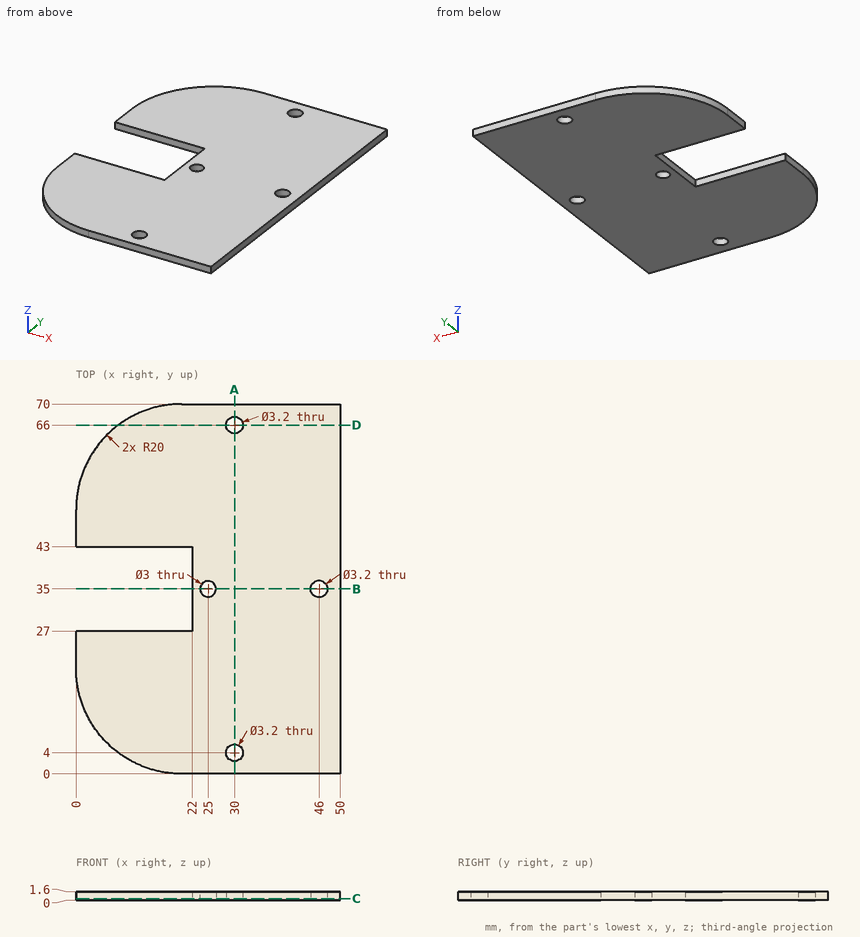
Study the drawing (mm; zero at the part's minimum x, y, z) and answer. Round coordinates to 2 decimals unless told otherwise and drop trailing zeros. Loops run counter-clockwise (first coordinate to the right, second up) from the corner with the lowest first, then second, coordinate; pieces in that order, holes last.
Q1. Section B-B, the plane y = 35 is taken. Determine the outline of the cut face in (x, z), then the cut area to 3 significant figures.
Q2. Section D-D, the plane y = 66 is taken. Determine the outline of the cut face in (x, z).
Q3. Section A-A, the plane x = 30 is taken. Determine the outline of the cut face in (y, z), then the cut area to 3 significant figures.
Q4. Find the intervals of material crossed by line 1 (Y direction, x = 30, z = 0.4); line 2 (Y direction, x = 19.5, z = 0.9); line 3 (X direction, y = 34, z = 1), in increasing order.
Q5. Section C-C, the plane z = 0.3 is taken. Determine the outline of the cut face in (x, y).
Q6. Given pin 1 Ø1.8 at (x, y) = (25, 35) entering from -Z, flat-ended and moving along its own axis, determine where the tip first touches the part or whether it passes through.
Completed:
1. outline: (22, 0) - (23.5, 0) - (23.5, 1.6) - (22, 1.6) - close; (26.5, 0) - (44.4, 0) - (44.4, 1.6) - (26.5, 1.6) - close; (47.6, 0) - (50, 0) - (50, 1.6) - (47.6, 1.6) - close
1. area: 34.9 mm2
2. outline: (8, 0) - (28.4, 0) - (28.4, 1.6) - (8, 1.6) - close; (31.6, 0) - (50, 0) - (50, 1.6) - (31.6, 1.6) - close
3. outline: (0, 0) - (2.4, 0) - (2.4, 1.6) - (0, 1.6) - close; (5.6, 0) - (64.4, 0) - (64.4, 1.6) - (5.6, 1.6) - close; (67.6, 0) - (70, 0) - (70, 1.6) - (67.6, 1.6) - close
3. area: 102 mm2
4. line 1: y = 0 to 2.4, 5.6 to 64.4, 67.6 to 70
4. line 2: y = 0.01 to 27, 43 to 69.99
4. line 3: x = 22 to 23.88, 26.12 to 44.75, 47.25 to 50
5. outline: (0, 20) arc R20 ccw to (20, 0) - (50, 0) - (50, 70) - (20, 70) arc R20 ccw to (0, 50) - (0, 43) - (22, 43) - (22, 27) - (0, 27) - close; hole circle Ø3 at (25, 35); hole circle Ø3.2 at (30, 4); hole circle Ø3.2 at (30, 66); hole circle Ø3.2 at (46, 35)
6. pin 1: passes through
